Drawing for the job (mm, zero at the part's lowest x, y, z). Round coordinates to 2 decimals unless told otherwise and drop trailing zeros. Loops run counter-clockwise (first coordinate to the right, second up) from the corner with the lowest first, then second, coordinate; pieces in that order, holes last. Notation, with made-up numbers: M 14,30 L 65,30 A6 ccw 65,39 Z; hole C 83.5,-22 d5. An arc over 180 degrees is marked long. Answer in a Markdown table with one row per item.
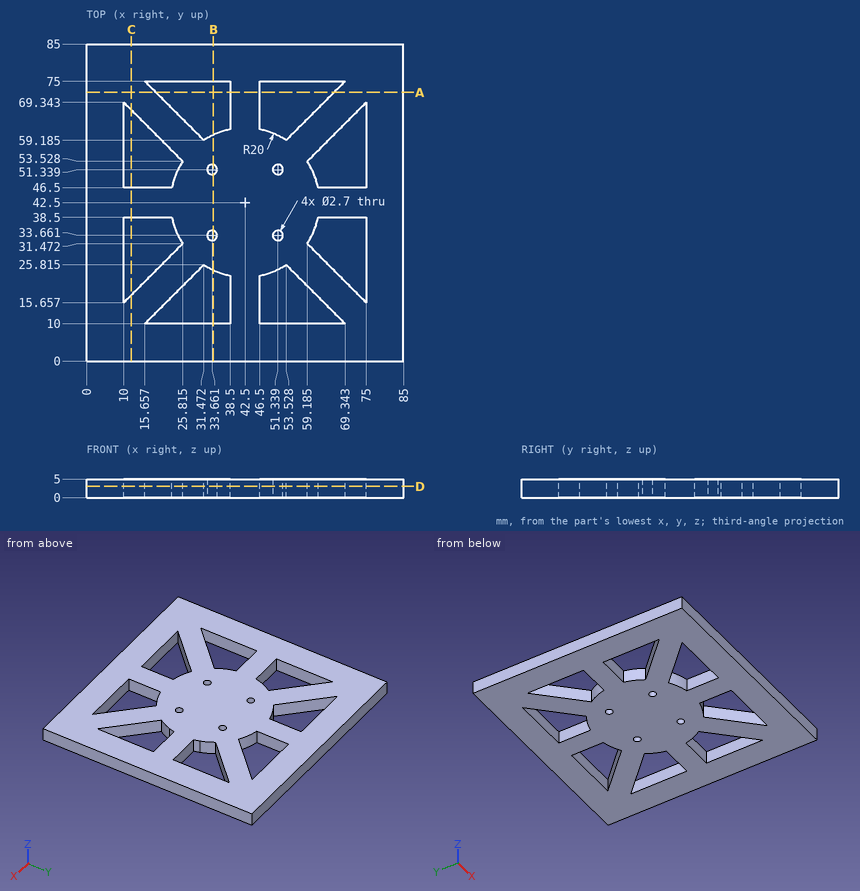
1. Saw through at C-C (x = 12). Write the cut outline in (y, z), and give its area (3 significant figures).
Verdict:
| item | result |
|---|---|
| outline | M 0,0 L 17.66,0 L 17.66,5 L 0,5 Z; M 38.5,0 L 46.5,0 L 46.5,5 L 38.5,5 Z; M 67.34,0 L 85,0 L 85,5 L 67.34,5 Z |
| area | 217 mm² |
2. Saw through at B-B (x = 34). Write the cut outline in (y, z).
Verdict:
| item | result |
|---|---|
| outline | M 0,0 L 10,0 L 10,5 L 0,5 Z; M 24.4,0 L 32.35,0 L 32.35,5 L 24.4,5 Z; M 34.97,0 L 50.03,0 L 50.03,5 L 34.97,5 Z; M 52.65,0 L 60.6,0 L 60.6,5 L 52.65,5 Z; M 75,0 L 85,0 L 85,5 L 75,5 Z |
3. Saw through at A-A (y = 72). Write the cut outline in (x, z).
Verdict:
| item | result |
|---|---|
| outline | M 0,0 L 18.66,0 L 18.66,5 L 0,5 Z; M 38.5,0 L 46.5,0 L 46.5,5 L 38.5,5 Z; M 66.34,0 L 85,0 L 85,5 L 66.34,5 Z |
4. Wall check: probe 1 along Y at (x, z) = (24.5, 2.8); probe 2 along Y at (x, z) = (53.5, 1.5); probe 3 along X at (y, z) = (25, 2.65). Give the ranges that are in metal, low to high.
Verdict:
| item | result |
|---|---|
| probe 1 | y = 0 to 10, 18.84 to 30.16, 33.78 to 51.22, 54.84 to 66.16, 75 to 85 |
| probe 2 | y = 0 to 10, 25.8 to 59.2, 75 to 85 |
| probe 3 | x = 0 to 10, 19.34 to 30.66, 32.82 to 52.18, 54.34 to 65.66, 75 to 85 |
5. Pin check, flat tip, straight feed: pin 1 (2 mm diameter, centred on x = 51.34, y = 33.66, fed in from +Z). Stop position of the tip, or through.
Verdict:
| item | result |
|---|---|
| pin 1 | passes through |
6. Saw through at D-D (z = 3). State how many separate pieces and enclosed holes the cut face has, and give its area (3 significant figures).
Verdict:
| item | result |
|---|---|
| separate pieces | 1 |
| enclosed holes | 12 |
| area | 5,410 mm² |
